Verification items for the finished model (mm, model axes). Face numbers are marked on the shaded views. Round coordinates to 2 decimals unless told otherwise and drop trailing zeros. Write each loop counter-clockwise with the first axis right and the second up, starting at its lowest first coordinate (ties: lowest second). Pieces come first, ordered by that corner, then holes. Notation, with made-up numbers: M 56.5,87.25 L 81.5,87.25 A27 cw 81.5,117.25 Z; hole C -25.75,84.25 d11. An arc over 180 degrees is marked long. Write each question's results on one line, items separated by ' | '.
from build123d import *

# Parameters (mm, degrees)
BOSS_EXTRUDE1_DEPTH     = 12.5
SKETCH2_R               = 40
BOSS_EXTRUDE2_DEPTH     = 80
BOSS_EXTRUDE3_DEPTH     = 12.5
CUT_EXTRUDE2_DEPTH      = 132.903899543
CUT_EXTRUDE2_DEPTH_BACK = 132.903899543
SKETCH6_R               = 32.5


with BuildPart() as part:
    # Sketch1 → Boss-Extrude1 (new body)
    with BuildSketch(Plane.XY):
        with BuildLine():
            Line((-30, -48), (30, -48))
            ThreePointArc((30, -48), (80.813999827, 0), (30, 48))
            Line((30, 48), (-30, 48))
            Line((-30, 48), (-30, -48))
        make_face()
    extrude(amount=BOSS_EXTRUDE1_DEPTH)

    # Sketch2 → Boss-Extrude2 (add)
    with BuildSketch(Plane.XY.offset(12.5)):
        with Locations((20, 0)):
            Circle(SKETCH2_R)
    extrude(amount=BOSS_EXTRUDE2_DEPTH)

    # Sketch3 → Boss-Extrude3 (add)
    with BuildSketch(Plane.XY.offset(92.5)):
        with BuildLine():
            Line((-30, 48), (-30, -48))
            Line((-30, -48), (30, -48))
            ThreePointArc((30, -48), (80.813999827, 0), (30, 48))
            Line((30, 48), (-30, 48))
        make_face()
    extrude(amount=BOSS_EXTRUDE3_DEPTH)

    # Sketch6 → Cut-Extrude2 (cut, two sides: drawn at the far end of the back side and taken through both)
    with BuildSketch(Plane.XY.offset(12.5).offset(-CUT_EXTRUDE2_DEPTH_BACK)):
        with Locations((20, 0)):
            Circle(SKETCH6_R)
    extrude(amount=CUT_EXTRUDE2_DEPTH + CUT_EXTRUDE2_DEPTH_BACK, mode=Mode.SUBTRACT)


solid = part.part
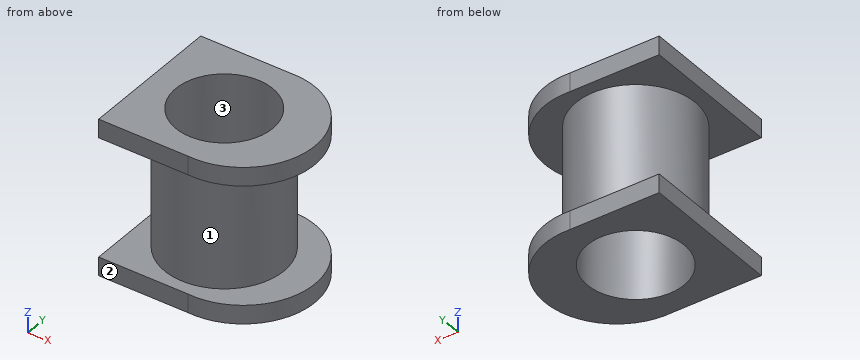
1) Sectioned sample at A-A, the plane x = 20. Record the cut outline in (y, z), and give its area (4 significant figures).
Calculated:
outline: M -48,0 L -32.5,0 L -32.5,105 L -48,105 L -48,92.5 L -40,92.5 L -40,12.5 L -48,12.5 Z; M 32.5,0 L 48,0 L 48,12.5 L 40,12.5 L 40,92.5 L 48,92.5 L 48,105 L 32.5,105 Z | area: 1,975 mm²
2) Sectioned sample at C-C, the plane z = 43.5. Record the cut outline in (x, y).
Calculated:
outline: C 20,0 d80; hole C 20,0 d65
3) Sectioned sample at D-D, the plane y = 36.5. Record the cut outline in (x, z).
Calculated:
outline: M -30,0 L 64.03,0 L 64.03,12.5 L 36.36,12.5 L 36.36,92.5 L 64.03,92.5 L 64.03,105 L -30,105 L -30,92.5 L 3.64,92.5 L 3.64,12.5 L -30,12.5 Z
4) Material ranges on line 1 (Z direction, x = -19, y = 36); line 2 (Y direction, x = 20, z = 71.5); line 3 (X direction, y = 23.5, z = 67), recorded low to high. Write a range as [from, to].
Calculated:
line 1: z = [0, 12.5], [92.5, 105] | line 2: y = [-40, -32.5], [32.5, 40] | line 3: x = [-12.37, -2.45], [42.45, 52.37]
5) Draft check along X on the marked faces 1, 2 and 3. Enter one of: pulls with the +X half, pulls with the -X half, needs draft (parallel to the pull), parting line crosses it, or undercut.
Calculated:
face 1: parting line crosses it | face 2: needs draft | face 3: undercut
6) Depth check by flat-ended pin: P1, Ø4, axis at x = -13.5, z = 3.5, coming from the -Y side; P2, Ø1, axis at x = 48.5, z = 24.5, coming from the -Y side; P3, Ø8, axis at x = -6, y = -3.5, coming from the +Z side; P4, Ø12, axis at y = -16.5, z = 66.5, coming from the +X side. Enter the tip coordinate at first touch or a pass-through.
Calculated:
P1: stops at y = -48 | P2: stops at y = -28.57 | P3: passes through | P4: stops at x = 58.6
7) Sectioned sample at B-B, the plane y = -17. Record the cut outline in (x, z).
Calculated:
outline: M -30,0 L -7.7,0 L -7.7,105 L -30,105 L -30,92.5 L -16.21,92.5 L -16.21,12.5 L -30,12.5 Z; M 47.7,0 L 77.71,0 L 77.71,12.5 L 56.21,12.5 L 56.21,92.5 L 77.71,92.5 L 77.71,105 L 47.7,105 Z
